from build123d import *

# Parameters (mm, degrees)
SKETCH1_W           = 38.4
SKETCH1_H           = 73
BOSS_EXTRUDE1_DEPTH = 5
SKETCH4_W           = 5
SKETCH4_H           = 25
BOSS_EXTRUDE3_DEPTH = 10
SKETCH5_R           = 1.6
CUT_EXTRUDE1_DEPTH  = 25
SKETCH6_W           = 5
SKETCH6_H           = 15
CUT_EXTRUDE2_DEPTH  = 5.9
SKETCH8_W           = 5
SKETCH8_H           = 73
CUT_EXTRUDE3_DEPTH  = 10
SKETCH9_R           = 0.975
CUT_EXTRUDE4_DEPTH  = 13


with BuildPart() as part:
    # Sketch1 → Boss-Extrude1 (new body)
    with BuildSketch(Plane.XY):
        Rectangle(SKETCH1_W, SKETCH1_H)
    extrude(amount=BOSS_EXTRUDE1_DEPTH)

    # Sketch4 → Boss-Extrude3 (add)
    with BuildSketch(Plane.ZY.offset(19.2)):
        with Locations((2.5, 0)):
            Rectangle(SKETCH4_W, SKETCH4_H)
    extrude(amount=BOSS_EXTRUDE3_DEPTH)

    # Sketch5 → Cut-Extrude1 (cut)
    with BuildSketch(Plane.XY.offset(5)):
        with Locations((-18.427514421, 6.717514421)):
            Circle(SKETCH5_R)
        with Locations((-6.053145751, 5.656854249)):
            Circle(SKETCH5_R)
        with Locations((-17.366854249, -5.656854249)):
            Circle(SKETCH5_R)
        with Locations((-4.992485579, -6.717514421)):
            Circle(SKETCH5_R)
    extrude(amount=-CUT_EXTRUDE1_DEPTH, mode=Mode.SUBTRACT)

    # Sketch6 → Cut-Extrude2 (cut)
    with BuildSketch(Plane.ZY.offset(19.2)):
        with Locations((2.5, 29)):
            Rectangle(SKETCH6_W, SKETCH6_H)
        with Locations((2.5, -29)):
            Rectangle(SKETCH6_W, SKETCH6_H)
    extrude(amount=-CUT_EXTRUDE2_DEPTH, mode=Mode.SUBTRACT)

    # Sketch8 → Cut-Extrude3 (cut)
    with BuildSketch(Plane(origin=(0, 0, 0), x_dir=(-1, 0, 0), z_dir=(0, 0, -1))):
        with Locations((-16.7, 0)):
            Rectangle(SKETCH8_W, SKETCH8_H)
    extrude(amount=-CUT_EXTRUDE3_DEPTH, mode=Mode.SUBTRACT)

    # Sketch9 → Cut-Extrude4 (cut)
    with BuildSketch(Plane(origin=(0, 0, 0), x_dir=(-1, 0, 0), z_dir=(0, 0, -1))):
        with Locations((3.3, 31.5)):
            Circle(SKETCH9_R)
        with Locations((3.3, -31.5)):
            Circle(SKETCH9_R)
    extrude(amount=-CUT_EXTRUDE4_DEPTH, mode=Mode.SUBTRACT)


solid = part.part
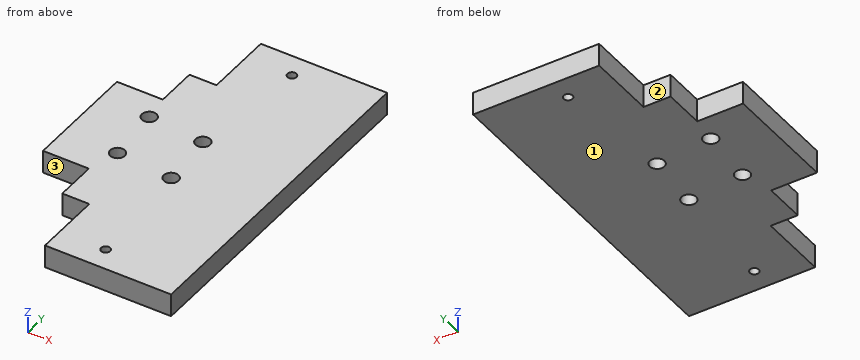
Could you check a few things on this model? Use its own coordinates, in mm. Face numbers are marked on the shaded views. A direction names the side the tool comes from. Coordinates: 2 decimals unless noted, no trailing zeros. Order: outer loops, then holes, each group sorted by start corner. A loop starts at its lowest first (then second) coordinate and runs counter-clockwise, first axis right, second up. Notation, with made-up numbers: (1, -35) -> (47, -35) arc R9 cw to (47, -22) -> close; hole circle Ø2 at (72, 15.5). An arc over 180 degrees is marked (long way). One line per item, written item: value. Start each with the question number.
1) Imagine slicing it at B-B on z = 3.8. List the corners of the cut face in (x, y) for me (3 decimals).
2) Imagine slicing it at C-C on y = -13.5. List the corners of the cut face in (x, z) for me, plus the area to 3 significant figures.
3) Imagine slicing it at A-A on y = -31.5. List the corners of the cut face in (x, z) for me (3 decimals).
4) If I drill on L1, parallel to Y at x = -3.3, z = 1.05 (3 decimals); L2, parallel to X at y = -7, z = 3.6; L3, parallel to Y at x = -17, z = 1.05, over which ranges is the centre line in solid material (lowest first)? Write a range as [from, to].
5) I'm going to push flat-ended pins straight in: pin 1 (1.8 mm diameter, centred on x = -3.3, y = -31.5, fed in from +Z); pin 2 (2.5 mm diameter, centred on x = -15, z = 3.5, fed in from -Y); pin 3 (2.5 mm diameter, centred on y = 16, z = 3, fed in from -X). Where does each tip first touch, or does it pass through?
6) Which directions (+Z, -Z, +X, -X, +Y, -Y) give clear straight access to the entire face, cutting with the end or side of a thin tool? Please do the marked faces 1, 2 and 3.
Answer list:
1. outline: (-29.2, -12.5) -> (-19.2, -12.5) -> (-19.2, -21.5) -> (-13.3, -21.5) -> (-13.3, -36.5) -> (14.2, -36.5) -> (14.2, 36.5) -> (-13.3, 36.5) -> (-13.3, 21.5) -> (-19.2, 21.5) -> (-19.2, 12.5) -> (-29.2, 12.5) -> close; hole circle Ø3.2 at (-18.428, 6.718); hole circle Ø3.2 at (-17.367, -5.657); hole circle Ø3.2 at (-6.053, 5.657); hole circle Ø3.2 at (-4.992, -6.718); hole circle Ø1.95 at (-3.3, -31.5); hole circle Ø1.95 at (-3.3, 31.5)
2. outline: (-19.2, 0) -> (14.2, 0) -> (14.2, 5) -> (-19.2, 5) -> close
2. area: 167 mm2
3. outline: (-13.3, 0) -> (-4.275, 0) -> (-4.275, 5) -> (-13.3, 5) -> close; (-2.325, 0) -> (14.2, 0) -> (14.2, 5) -> (-2.325, 5) -> close
4. L1: y = [-36.5, -32.475], [-30.525, 30.525], [32.475, 36.5]
4. L2: x = [-29.2, -18.24], [-16.5, -6.57], [-3.42, 14.2]
4. L3: y = [-21.5, -7.21], [-4.1, 5.99], [7.44, 21.5]
5. pin 1: passes through
5. pin 2: stops at y = -21.5
5. pin 3: stops at x = -19.2
6. face 1: -Z, +X, -X, +Y, -Y
6. face 2: +Z, -Z, -X, +Y
6. face 3: +Z, -Z, -X, -Y
